```python
from build123d import *

# Parameters (mm, degrees)
SKETCH1_R           = 9.5
COUPLING_BODY_DEPTH = 24.6
F_5MM_HOLE_REACH    = 26.6
SKETCH2_R           = 2.5
SKETCH3_R           = 4
F_8_MM_HOLE_DEPTH   = 17.25


with BuildPart() as part:
    # Sketch1 → coupling body (new body)
    with BuildSketch(Plane(origin=(0, 0, 0), x_dir=(1, 0, 0), z_dir=(0, 1, 0))):
        Circle(SKETCH1_R)
    extrude(amount=COUPLING_BODY_DEPTH)

    # Sketch2 → 5mm hole (cut, up to next)
    with BuildSketch(Plane(origin=(0, 24.6, 0), x_dir=(1, 0, 0), z_dir=(0, 1, 0)), mode=Mode.PRIVATE) as f_5mm_hole_sk1:
        Circle(SKETCH2_R)
    f_5mm_hole_tool1 = extrude(f_5mm_hole_sk1.sketch, amount=-F_5MM_HOLE_REACH, mode=Mode.PRIVATE) & part.part
    add(f_5mm_hole_tool1.solids().sort_by_distance((0, 24.6, 0))[0], mode=Mode.SUBTRACT)

    # Sketch3 → 8 mm hole (cut)
    with BuildSketch(Plane.XZ):
        Circle(SKETCH3_R)
    extrude(amount=-F_8_MM_HOLE_DEPTH, mode=Mode.SUBTRACT)


solid = part.part
```
Check sheet for the modelled part. Datum: model origin and axes. Units: mm. Round coordinates to 2 decimals unless told otherwise and drop trailing zeros. Order: outer loops, then holes, each group sorted by start corner. A loop starts at its lowest first (then second) coordinate and runs counter-clockwise, first axis right, second up.
1) Section check A-A (x = 0). Record the boundary of the cut face in (y, z).
2) Section check C-C (y = 10.5). Record the boundary of the cut face in (x, z).
3) Scan lines: line 1 (Z direction, x = 0, y = 19); line 2 (Z direction, x = 0, y = 10). Record each from-to range of solid material in increasing order.
4) Mould release check, pull along X, two halves, no side actions. Record for faces 1 (the cylindrical face through (4.38, 12.13, 8.43)), 2 (the flat face through (2, 17.25, 2)), 3 (the flat face through (4, 0, 2)), 4 (the cylindrical face through (-0.867, 8.504, -3.905)): +X half, -X half, draft (parallel to the pull), parting line (faces both ways), or undercut.
5) Go/stop test with flat-tipped pins: pin 1 Ø4 at (x, z) = (0, 0) entering from -Y; pin 2 Ø3 at (y, z) = (14, 2) entering from +X; pin 3 Ø6 at (x, y) = (5.5, 18) entering from +Z; pin 4 Ø4 at (x, y) = (5.5, 18) entering from +Z. Record where each tip stops, or that it passes through.
6) Section check B-B (z = 0). Record the boundary of the cut face in (x, y), and give its area (3 significant figures).
7) Section check D-D (y = 22.25). Record the boundary of the cut face in (x, z), and give its area (3 significant figures).
Result:
1. outline: (0, -9.5) - (24.6, -9.5) - (24.6, -2.5) - (17.25, -2.5) - (17.25, -4) - (0, -4) - close; (0, 4) - (17.25, 4) - (17.25, 2.5) - (24.6, 2.5) - (24.6, 9.5) - (0, 9.5) - close
2. outline: circle Ø19 at (0, 0); hole circle Ø8 at (0, 0)
3. line 1: z = -9.5 to -2.5, 2.5 to 9.5
3. line 2: z = -9.5 to -4, 4 to 9.5
4. face 1: parting line
4. face 2: undercut
4. face 3: draft
4. face 4: undercut
5. pin 1: passes through
5. pin 2: stops at x = 9.49
5. pin 3: stops at z = 9.17
5. pin 4: stops at z = 8.83
6. outline: (-9.5, 0) - (-4, 0) - (-4, 17.25) - (-2.5, 17.25) - (-2.5, 24.6) - (-9.5, 24.6) - close; (2.5, 17.25) - (4, 17.25) - (4, 0) - (9.5, 0) - (9.5, 24.6) - (2.5, 24.6) - close
6. area: 293 mm2
7. outline: circle Ø19 at (0, 0); hole circle Ø5 at (0, 0)
7. area: 264 mm2
